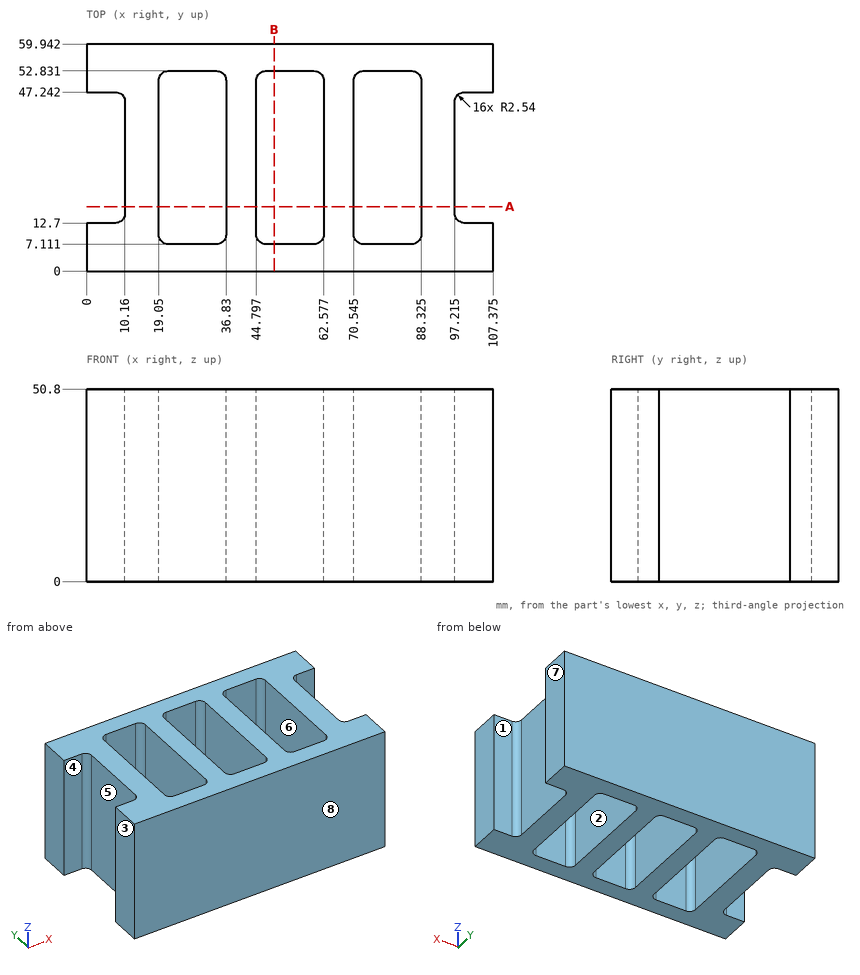
For this review, use the dimensioned drawing (mm, ordinates from the lowest corner) and the shaded views. A direction names the side the tool comes from. Give positions to 0.01 mm unless a question says otherwise; leave off trailing zeros. Write each loop counter-clockwise with the first axis right and the second up, starting at its lowest first coordinate (ties: lowest second). Pieces come first, ordered by that corner, then holes. Notation, with made-up numbers: M 50.5,61 L 89.5,61 A25 ccw 89.5,84 Z; hole C -19.75,26 d5. An arc over 180 degrees is marked long. Answer as a JSON object with one key per item and string values. Group by question number.
1) We need section B-B (x = 49.5). Give the boundary of the cut face in (y, z).
2) Clearance check with flat-ended pins moving along their axes: pin 1 Ø23.5 at (y, z) = (25.5, 32.5) entering from -X; pin 2 Ø23.5 at (y, z) = (34.5, 22) entering from +X; pin 3 Ø12 at (y, z) = (32, 26.5) entering from +X (1 decimal). State where each tip first meets the part, or that it passes through.
3) Tool access review of the marked faces 1, 2, 3 and 4: name each direction out of +Z, -Z, +X, -X, +Y, -Y from which nothing blocks a thin tool from reaching the whole face with its end or side.
4) Mouldability with a two-part tool opening along Y and no side actions: class the marked faces 5, 6, 7 and 8 as released by +Y, released by -Y, zero draft, split by the parting line, or undercut.
5) We need section A-A (y = 17). Count the separate pieces of the cut face and the enclosed holes in it, and give its area (3 significant figures).
6) For line 1 along Y through (x, z) = (58, 35); line 2 along Y through (x, z) = (7.5, 25), list the stretches that pass through material, from the lowest coordinate up.
Answer key:
{
 "1": {"outline": "M 0,0 L 7.11,0 L 7.11,50.8 L 0,50.8 Z; M 52.83,0 L 59.94,0 L 59.94,50.8 L 52.83,50.8 Z"},
 "2": {"pin 1": "stops at x = 9.68", "pin 2": "stops at x = 97.74", "pin 3": "stops at x = 97.2"},
 "3": {"face 1": "+Z, -Z, +X", "face 2": "+Z, -Z", "face 3": "+Z, -Z, -X, +Y, -Y", "face 4": "+Z, -Z, -X"},
 "4": {"face 5": "undercut", "face 6": "undercut", "face 7": "zero draft", "face 8": "released by -Y"},
 "5": {"separate pieces": "4", "enclosed holes": "0", "area": "1,710 mm²"},
 "6": {"line 1": "y = 0 to 7.11, 52.83 to 59.94", "line 2": "y = 0 to 12.7, 47.24 to 59.94"}
}
